Check sheet for the modelled part. Datum: model origin and axes. Units: mm. Round coordinates to 2 decimals unless told otherwise and drop trailing zeros. Order: outer loops, then holes, each group sorted by start corner. A loop starts at its lowest first (then second) coordinate and runs counter-clockwise, first axis right, second up. Notation, with made-up numbers: (-32, 88.5) -> (-13, 88.5) arc R32 ccw to (-13, 118.5) -> close; hole circle Ø4 at (36, 63.5). An arc over 180 degrees is marked (long way). Answer in a Markdown table with one row per item.
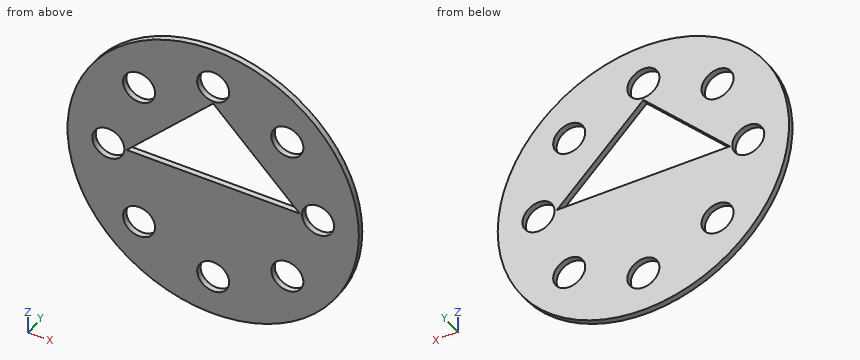
from build123d import *

# Parameters (mm, degrees)
SKETCH_1_R               = 25
EXTRUDE_2_DEPTH          = 1
SKETCH_2_R               = 1.5
CUT_EXTRUDE_1_DEPTH      = 1
PATTERN_CIRCULAR_1_COUNT = 8
CUT_EXTRUDE_2_DEPTH      = 1
EXTRUDE_3_DEPTH          = 1
SKETCH_5_R               = 25
EXTRUDE_5_DEPTH          = 2
SKETCH_6_R               = 1.5
CUT_EXTRUDE_3_DEPTH      = 2
PATTERN_CIRCULAR_2_COUNT = 8
SKETCH_7_R               = 25
EXTRUDE_6_DEPTH          = 2
SKETCH_8_R               = 2.75
CUT_EXTRUDE_4_DEPTH      = 2
PATTERN_CIRCULAR_3_COUNT = 8
EXTRUDE_8_DEPTH          = 2
SKETCH_11_R              = 25
CUT_EXTRUDE_6_DEPTH      = 4


with BuildPart() as part:
    # 草图1 → 凸台-拉伸2 (new body)
    with BuildSketch(Plane(origin=(0, 0, 0), x_dir=(1, 0, 0), z_dir=(0, 1, 0))):
        Circle(SKETCH_1_R)
    extrude(amount=EXTRUDE_2_DEPTH)

    # 草图2 → 切除-拉伸1 (cut)
    with BuildSketch(Plane(origin=(0, 1, 0), x_dir=(1, 0, 0), z_dir=(0, 1, 0))):
        with Locations((18, 0)):
            Circle(SKETCH_2_R)
    cut_extrude_1 = extrude(amount=-CUT_EXTRUDE_1_DEPTH, mode=Mode.SUBTRACT)

    # 阵列(圆周)1: 切除-拉伸1 ×8 about axis
    pattern_circular_1_axis = Axis((0, 0, 0), (0, 1, 0))
    for i in range(1, PATTERN_CIRCULAR_1_COUNT):
        add(cut_extrude_1.rotate(pattern_circular_1_axis, i * 360 / PATTERN_CIRCULAR_1_COUNT), mode=Mode.SUBTRACT)

    # 草图3 → 切除-拉伸2 (cut)
    with BuildSketch(Plane(origin=(0, 1, 0), x_dir=(1, 0, 0), z_dir=(0, 1, 0))):
        Polygon((-15.202795796, 0), (15.202795796, 0), (0, -15.202795796), align=None)
    extrude(amount=-CUT_EXTRUDE_2_DEPTH, mode=Mode.SUBTRACT)

    # 草图4 → 凸台-拉伸3 (add)
    with BuildSketch(Plane(origin=(0, 1, 0), x_dir=(1, 0, 0), z_dir=(0, 1, 0))):
        Polygon((0, -14.849242405), (14.849242405, 0), (15.202795796, 0), (0, -15.202795796), (-15.202795796, 0), (-14.849242405, 0), align=None)
    extrude(amount=-EXTRUDE_3_DEPTH)

    # 草图5 → 凸台-拉伸5 (add)
    with BuildSketch(Plane.XZ):
        Circle(SKETCH_5_R)
    extrude(amount=EXTRUDE_5_DEPTH)

    # 草图6 → 切除-拉伸3 (cut)
    with BuildSketch(Plane(origin=(0, 0, 0), x_dir=(1, 0, 0), z_dir=(0, 1, 0))):
        with Locations((18, 0)):
            Circle(SKETCH_6_R)
    cut_extrude_3 = extrude(amount=-CUT_EXTRUDE_3_DEPTH, mode=Mode.SUBTRACT)

    # 阵列(圆周)2: 切除-拉伸3 ×8 about axis
    pattern_circular_2_axis = Axis((0, 0, 0), (0, 1, 0))
    for i in range(1, PATTERN_CIRCULAR_2_COUNT):
        add(cut_extrude_3.rotate(pattern_circular_2_axis, i * 360 / PATTERN_CIRCULAR_2_COUNT), mode=Mode.SUBTRACT)

    # 草图7 → 凸台-拉伸6 (add)
    with BuildSketch(Plane(origin=(0, 1, 0), x_dir=(1, 0, 0), z_dir=(0, 1, 0))):
        Circle(SKETCH_7_R)
        Polygon((-14.849242405, 0), (14.849242405, 0), (0, -14.849242405), align=None, mode=Mode.SUBTRACT)
    extrude(amount=EXTRUDE_6_DEPTH)

    # 草图8 → 切除-拉伸4 (cut)
    with BuildSketch(Plane(origin=(0, 1, 0), x_dir=(1, 0, 0), z_dir=(0, 1, 0))):
        with Locations((18, 0)):
            Circle(SKETCH_8_R)
    cut_extrude_4 = extrude(amount=CUT_EXTRUDE_4_DEPTH, mode=Mode.SUBTRACT)

    # 阵列(圆周)3: 切除-拉伸4 ×8 about axis
    pattern_circular_3_axis = Axis((0, 0, 0), (0, 1, 0))
    for i in range(1, PATTERN_CIRCULAR_3_COUNT):
        add(cut_extrude_4.rotate(pattern_circular_3_axis, i * 360 / PATTERN_CIRCULAR_3_COUNT), mode=Mode.SUBTRACT)

    # 草图9 → 凸台-拉伸8 (add)
    with BuildSketch(Plane(origin=(0, 0, 0), x_dir=(1, 0, 0), z_dir=(0, 1, 0))):
        Polygon((-14.849242405, 0), (14.849242405, 0), (0, -14.849242405), align=None)
    extrude(amount=EXTRUDE_8_DEPTH)

    # 草图11 → 切除-拉伸6 (cut)
    with BuildSketch(Plane.XZ.offset(2)):
        Circle(SKETCH_11_R)
    extrude(amount=-CUT_EXTRUDE_6_DEPTH, mode=Mode.SUBTRACT)


solid = part.part
Item 1: Cross-section at D-D (z = -18). Record the boundary of the cut face in (x, y), and give its area (3 significant figures).
Result sheet:
| item | result |
|---|---|
| outline | (-17.35, 2) -> (-2.75, 2) -> (-2.75, 3) -> (-17.35, 3) -> close; (2.75, 2) -> (17.35, 2) -> (17.35, 3) -> (2.75, 3) -> close |
| area | 29.2 mm^2 |
Item 2: Cross-section at A-A (x = 4.5). Record the boundary of the cut face in (y, z), and give its area (3 significant figures).
Result sheet:
| item | result |
|---|---|
| outline | (2, -24.59) -> (3, -24.59) -> (3, 0) -> (2, 0) -> close; (2, 10.35) -> (3, 10.35) -> (3, 24.59) -> (2, 24.59) -> close |
| area | 38.8 mm^2 |
Item 3: Cross-section at C-C (y = 2.2). State how many separate pieces and enclosed holes the cut face has, and give its area (3 significant figures).
Result sheet:
| item | result |
|---|---|
| separate pieces | 1 |
| enclosed holes | 9 |
| area | 1,550 mm^2 |
Item 4: Cross-section at B-B (z = -11). Record the boundary of the cut face in (x, y), and give its area (3 significant figures).
Result sheet:
| item | result |
|---|---|
| outline | (-22.45, 2) -> (-14.87, 2) -> (-14.87, 3) -> (-22.45, 3) -> close; (-10.59, 2) -> (10.59, 2) -> (10.59, 3) -> (-10.59, 3) -> close; (14.87, 2) -> (22.45, 2) -> (22.45, 3) -> (14.87, 3) -> close |
| area | 36.3 mm^2 |
Item 5: Scan lines: line 1 (X direction, y = 2.2, z = -1); line 2 (X direction, y = 2.65, z = 14); line 3 (X direction, y = 2.6, z = -11.5). Record each from-to range of solid material in increasing order. Write a range as [from, to].
Result sheet:
| item | result |
|---|---|
| line 1 | x = [-24.98, -20.56], [-15.44, 15.44], [20.56, 24.98] |
| line 2 | x = [-20.71, -15.17], [-10.29, -0.85], [0.85, 10.29], [15.17, 20.71] |
| line 3 | x = [-22.2, -15.19], [-10.27, 10.27], [15.19, 22.2] |
